from build123d import *

# Parameters (mm, degrees)
SKETCH1_R               = 1.5
BOSS_EXTRUDE1_DEPTH     = 50
CUT_EXTRUDE1_DEPTH      = 2
CUT_EXTRUDE1_DEPTH_BACK = 50
SKETCH3_W               = 2
SKETCH3_H               = 4.5
CUT_EXTRUDE2_DEPTH      = 50
CUT_EXTRUDE2_DEPTH_BACK = 50
SKETCH4_R               = 0.8


with BuildPart() as part:
    # Sketch1 → Boss-Extrude1 (new body)
    with BuildSketch(Plane.XY):
        with Locations((0, 3.147273027)):
            Circle(SKETCH1_R)
    extrude(amount=BOSS_EXTRUDE1_DEPTH)

    # Sketch3 → Cut-Extrude1 (cut, two sides: drawn at the far end of the back side and taken through both)
    with BuildSketch(Plane(origin=(0, 0, 0), x_dir=(1, 0, 0), z_dir=(0, 1, 0)).offset(-CUT_EXTRUDE1_DEPTH_BACK)):
        with Locations((0, -48.75)):
            Rectangle(SKETCH3_W, SKETCH3_H)
        with Locations((0, -1.25)):
            Rectangle(SKETCH3_W, SKETCH3_H)
    extrude(amount=CUT_EXTRUDE1_DEPTH + CUT_EXTRUDE1_DEPTH_BACK, mode=Mode.SUBTRACT)

    # Sketch4 → Cut-Extrude2 (cut, two sides: drawn at the far end of the back side and taken through both)
    with BuildSketch(Plane(origin=(0, 0, 0), x_dir=(1, 0, 0), z_dir=(0, 1, 0)).offset(-CUT_EXTRUDE2_DEPTH_BACK)):
        with Locations(Location((0, -48, 0), (0, 0, 90))):
            Circle(SKETCH4_R)
        with Locations(Location((0, -2, 0), (0, 0, 90))):
            Circle(SKETCH4_R)
    extrude(amount=CUT_EXTRUDE2_DEPTH + CUT_EXTRUDE2_DEPTH_BACK, mode=Mode.SUBTRACT)


solid = part.part
Geometry check sheet. Reference: the model listing, model coordinates, mm. A direction names the side the tool comes from. Round coordinates to 2 decimals unless told otherwise and drop trailing zeros. Order: outer loops, then holes, each group sorted by start corner. A loop starts at its lowest first (then second) coordinate and runs counter-clockwise, first axis right, second up. Notation, with made-up numbers: M -16,40.25 L 10,40.25 A17 cw 10,65.25 Z; hole C -28.5,-29 d1. An arc over 180 degrees is marked long. Answer in a Markdown table with one row per item.
(1) Sectioned sample at A-A, the plane x = 0. Record the cut outline in (y, z).
Responses:
| item | result |
|---|---|
| outline | M 1.65,3.5 L 2,3.5 L 2,2.8 L 4.65,2.8 L 4.65,47.2 L 2,47.2 L 2,46.5 L 1.65,46.5 Z; M 2,0 L 4.65,0 L 4.65,1.2 L 2,1.2 Z; M 2,48.8 L 4.65,48.8 L 4.65,50 L 2,50 Z |
(2) Sectioned sample at C-C, the plane z = 48. Record the cut outline in (x, y), and give its area (3 significant figures).
Responses:
| item | result |
|---|---|
| outline | M -0.97,2 L -0.8,2 L -0.8,4.42 A1.5 ccw Z; M 0.8,2 L 0.97,2 A1.5 ccw 0.8,4.42 Z |
| area | 2.49 mm² |
(3) Draft check along X on faces 4 (the face through (-0.793, 3.305, 2.104)), 5 (the face through (0, 3, 50)), 6 (the face through (-0.195, 4.635, 24.65)). Enter one of: released by +X, released by -X, zero draft, split by the parting line, or undercut.
Responses:
| item | result |
|---|---|
| face 4 | undercut |
| face 5 | zero draft |
| face 6 | split by the parting line |
(4) Scan lines: probe 1 along X at (y, z) = (3.1, 48); probe 2 along Z at (x, y) = (-0.55, 2.55); probe 3 along Y at (x, z) = (-0.1, 34.5). Record each from-to range of solid material in increasing order. Write a range as from..to.
Responses:
| item | result |
|---|---|
| probe 1 | x = -1.5..-0.8, 0.8..1.5 |
| probe 2 | z = 0..1.42, 2.58..47.42, 48.58..50 |
| probe 3 | y = 1.65..4.64 |
(5) Sectioned sample at D-D, the plane z = 27.5. Record the cut outline in (x, y).
Responses:
| item | result |
|---|---|
| outline | C 0,3.15 d3 |
(6) Go/stop test with flat-tipped pins: P1, Ø1, axis at x = 0.5, z = 2, coming from the -Y side; P2, Ø1.8, axis at x = 0, z = 2, coming from the +Y side; P3, Ø1.5, axis at y = 4, z = 25.5, coming from the +X side. Record where each tip stops, or that it passes through.
Responses:
| item | result |
|---|---|
| P1 | stops at y = 2 |
| P2 | stops at y = 4.65 |
| P3 | stops at x = 1.5 |
(7) Sectioned sample at B-B, the plane y = 2.45. Record the cut outline in (x, z), and give its area (3 significant figures).
Responses:
| item | result |
|---|---|
| outline | M -1.33,0 L 1.33,0 L 1.33,50 L -1.33,50 Z; hole C 0,2 d1.6; hole C 0,48 d1.6 |
| area | 129 mm² |
(8) Tool access check on faces 1 (the face through (0, 2, 49)), 2 (the face through (-0.793, 3.305, 48.104)), 3 (the face through (0, 2, 1)). Record the directions out of +Z, -Z, +X, -X, +Y, -Y that give a thin tool (end or side, any length) a straight path to the whole face; none if there is none.
Responses:
| item | result |
|---|---|
| face 1 | +Z, +X, -X, -Y |
| face 2 | +Y, -Y |
| face 3 | -Z, +X, -X, -Y |
